For this review, take the finished solid that the model builds, in its own axes (mm). A direction names the side the tool comes from. Coordinates: 2 decimals unless noted, no trailing zeros. Order: outer loops, then holes, each group sorted by start corner. A loop starts at its lowest first (then second) coordinate and runs counter-clockwise, first axis right, second up. Notation, with made-up numbers: (48.25, -0.75) - (97.25, -0.75) arc R19 ccw to (97.25, 5.25) - close; hole circle Ø10 at (-7, 65). An arc over 180 degrees is marked (long way). One line per item, written item: value. Start each with the question number.
(1) Consider section A-A on x = 0. Write out the cut boundary in (y, z), then the cut area to 3 significant figures.
(2) Consider section C-C on y = -2.25. Write out the cut boundary in (x, z), then the cut area to 3 significant figures.
(3) Mouldability with a two-part tool opening along X and no side actions: class faces 1 (the cylindrical face through (-1.009, -1.602, 7.684)), 2 (the flat face through (5.7, -3.25, -4.6)), 3 (the cylindrical face through (-0.9, -0.8, -7.1)) as released by +X, released by -X, zero draft, split by the parting line, or undercut.
(4) Consider section D-D on x = 9.75. Write out the cut boundary in (y, z).
(5) For faces 4 (the flat face through (6, 0, 6)), 5 (the flat face through (6, 1.5, 6)), list the 3-axis set-ups (+Z, -Z, +X, -X, +Y, -Y) from which the entire face can be reached by the end or side of a thin tool; tool diameter is ignored.
(6) Consider section B-B on z = 0. Write out the cut boundary in (x, y).
(7) Clearance check with flat-ended pins moving along their axes: pin 1 (1 mm diameter, centred on y = 1, z = 3.5, fed in from +X); pin 2 (8 mm diameter, centred on x = -3.5, z = -5, fed in from +Y). State where each tip first meets the part, or that it passes through.
(8) To check wall thickness, follow line 1 along X through (y, z) = (0.1, 0); line 2 along Z through (x, y) = (0, -0.1); line 3 along X through (y, z) = (-2.6, 0.25). State the ranges of each line that lie inside material, in increasing order.
```python
from build123d import *

# Parameters (mm, degrees)
SKETCH1_R           = 13
BOSS_EXTRUDE1_DEPTH = 1.5
SKETCH2_R           = 7.75
BOSS_EXTRUDE2_DEPTH = 3.25
SKETCH3_R           = 7.1554
CUT_EXTRUDE1_DEPTH  = 5.75


with BuildPart() as part:
    # Sketch1 → Boss-Extrude1 (new body)
    with BuildSketch(Plane(origin=(0, 0, 0), x_dir=(1, 0, 0), z_dir=(0, 1, 0))):
        Circle(SKETCH1_R)
    extrude(amount=BOSS_EXTRUDE1_DEPTH)

    # Sketch2 → Boss-Extrude2 (add)
    with BuildSketch(Plane.XZ):
        Circle(SKETCH2_R)
    extrude(amount=BOSS_EXTRUDE2_DEPTH)

    # Sketch3 → Cut-Extrude1 (cut, through all)
    with BuildSketch(Plane(origin=(0, 1.5, 0), x_dir=(1, 0, 0), z_dir=(0, 1, 0))):
        Circle(SKETCH3_R)
    extrude(amount=-CUT_EXTRUDE1_DEPTH, mode=Mode.SUBTRACT)


solid = part.part
```
Geometry check:
1. outline: (-3.25, -7.75) - (0, -7.75) - (0, -13) - (1.5, -13) - (1.5, -7.16) - (-3.25, -7.16) - close; (-3.25, 7.16) - (1.5, 7.16) - (1.5, 13) - (0, 13) - (0, 7.75) - (-3.25, 7.75) - close
1. area: 21.4 mm^2
2. outline: circle Ø15.5 at (0, 0); hole circle Ø14.31 at (0, 0)
2. area: 27.8 mm^2
3. face 1: split by the parting line
3. face 2: zero draft
3. face 3: undercut
4. outline: (0, -8.6) - (1.5, -8.6) - (1.5, 8.6) - (0, 8.6) - close
5. face 4: -Y
5. face 5: +Z, -Z, +X, -X, +Y
6. outline: (-13, 0) - (-7.75, 0) - (-7.75, -3.25) - (-7.16, -3.25) - (-7.16, 1.5) - (-13, 1.5) - close; (7.16, -3.25) - (7.75, -3.25) - (7.75, 0) - (13, 0) - (13, 1.5) - (7.16, 1.5) - close
7. pin 1: stops at x = 12.65
7. pin 2: stops at y = 1.5
8. line 1: x = -13 to -7.16, 7.16 to 13
8. line 2: z = -7.75 to -7.16, 7.16 to 7.75
8. line 3: x = -7.75 to -7.15, 7.15 to 7.75
